Geometry check sheet. Reference: the model listing, model coordinates, mm. Round coordinates to 2 decimals unless told otherwise and drop trailing zeros. Write each loop counter-clockwise with the first axis right and the second up, starting at its lowest first coordinate (ties: lowest second). Pieces come first, ordered by that corner, then holes. Notation, with made-up numbers: (-15.75, 72.25) -> (37.25, 72.25) arc R8 cw to (37.25, 82.25) -> close; hole circle Ø6 at (-19.5, 19). An arc over 180 degrees is marked (long way). Use a Markdown table: item, result.
```python
from build123d import *

# Parameters (mm, degrees)
F0_R     = 50.8
F1_DEPTH = 19.05
F2_SIZE2 = 11.76551
F2_SIZE  = 19.04999
F3_SIZE  = 5.08


# Not quite as in the source:
# - a fillet or chamfer is up to 0.001 mm smaller than in the source, because OpenCascade refuses the exact size


with BuildPart() as f1:
    # F0 (on Top) → F1 (new body)
    with BuildSketch(Plane.XY):
        Polygon((0, 108.0326526607), (-102.7451582856, 33.3839256196), (-63.5, -87.4002519499), (63.5, -87.4002519499), (102.7451582856, 33.3839256196), align=None)
        Circle(F0_R, mode=Mode.SUBTRACT)
    extrude(amount=F1_DEPTH)

    # F2 (size 19.05 and 11.7655197988 in the source; OpenCascade refuses exactly that, so slightly less here)
    f2_edges = [f1.edges().sort_by_distance(p)[0] for p in [
        (0, -87.400252, 19.05),
        (83.122579, -27.008163, 19.05),
        (51.372579, 70.708289, 19.05),
        (-51.372579, 70.708289, 19.05),
        (-83.122579, -27.008163, 19.05),
    ]]
    chamfer(f2_edges, length=F2_SIZE, length2=F2_SIZE2)

    # F3
    f3_edges = [f1.edges().sort_by_distance(p)[0] for p in [
        (-50.8, 0, 0),
    ]]
    chamfer(f3_edges, length=F3_SIZE)


solid = f1.part
```
(1) Gauge pin test, flat ends, axial feed: pin 1 Ø1.5 at (x, z) = (29, 14.5) entering from +Y; pin 2 Ø10 at (y, z) = (39.5, 15) entering from +X; pin 3 Ø1 at (x, z) = (2, 17) entering from +Y. Record the tip position at first contact, or that the pin passes through.
A:
| item | result |
|---|---|
| pin 1 | stops at y = 76.68 |
| pin 2 | stops at x = 87.22 |
| pin 3 | stops at y = 94.13 |
(2) Release check for a two-part mould opening along X. For faces 1 (the face through (-77.724, -24.319, 9.658)), 2 (the face through (77.175, -26.01, 9.658)), 3 (the face through (-47, -32, 0)), 4 (the face through (-11.012, -49.592, 11.967)) record: +X half, -X half, draft (parallel to the pull), parting line (faces both ways), or undercut.
A:
| item | result |
|---|---|
| face 1 | -X half |
| face 2 | +X half |
| face 3 | draft |
| face 4 | undercut |
(3) Thickness scan on line 1 (Y direction, x = 18, z = 9.5); line 2 (Y direction, x = -35, z = 11.25); line 3 (X direction, y = 31, z = 13.5). Record the ranges inside material, lowest first.
A:
| item | result |
|---|---|
| line 1 | y = -81.53 to -47.5, 47.5 to 87.7 |
| line 2 | y = -80.45 to -36.82, 36.82 to 74.02 |
| line 3 | x = -91.84 to -40.24, 40.24 to 91.84 |
(4) Section check B-B on z = 8.5. Record the cut outline in (x, y), plus the area to 3 significant figures.
A:
| item | result |
|---|---|
| outline | (-96.57, 31.38) -> (-59.69, -82.15) -> (59.69, -82.15) -> (96.57, 31.38) -> (0, 101.54) -> close; hole circle Ø101.6 at (0, 0) |
| area | 16,400 mm2 |
